CAD build for the part. Positions are in the model's coordinates, mm. Coordinates: 2 decimals unless noted, no trailing zeros. Loops run counter-clockwise (first coordinate to the right, second up) from the corner with the lowest first, then second, coordinate; pieces in that order, holes last. Notation, with made-up numbers: (18.5, 83) - (35.5, 83) arc R12 ccw to (35.5, 103) - close; hole circle Ø11 at (-24.75, 37.25). An arc over 180 degrees is marked (long way). Put each result on its own line as item: value.
```python
from build123d import *

# Parameters (mm, degrees)
CUT_EXTRUDE_1_DEPTH      = 10
PATTERN_CIRCULAR_2_COUNT = 28
SKETCH_3_R               = 5
CUT_EXTRUDE_2_DEPTH      = 26.454679665


with BuildPart() as part:
    # 草图1 → 旋转1 (revolve)
    with BuildSketch(Plane.XY, mode=Mode.PRIVATE) as revolve_1_sk:
        Polygon((-4.537524852, 10.783302268), (-14.537524852, 10.783302268), (-14.537524852, 1.783302268), (-15.787524852, 1.783302268), (-15.787524852, -3.216697732), (-3.287524852, -3.216697732), (-3.287524852, 1.783302268), (-4.537524852, 1.783302268), align=None)
    revolve(revolve_1_sk.sketch.rotate(Axis((-37.951477077, -3.216697732, 0), (1, 0, 0)), 90), axis=Axis((-37.951477077, -3.216697732, 0), (1, 0, 0)))

    # 草图2 → 切除-拉伸1 (cut)
    with BuildSketch(Plane.ZY.offset(14.537524852)):
        with BuildLine():
            Line((0.390901935, 85.320682721), (-0.569796452, 10.771702176))
            ThreePointArc((-0.569796452, 10.771702176), (0.830427689, 9.255687358), (2.419277547, 10.572685726))
            Line((2.419277547, 10.572685726), (11.35038276, 84.590986174))
            Line((11.35038276, 84.590986174), (21.256411219, 233.371913604))
            Line((21.256411219, 233.371913604), (10.296930394, 234.10161015))
            Line((10.296930394, 234.10161015), (0.390901935, 85.320682721))
        make_face()
    cut_extrude_1 = extrude(amount=-CUT_EXTRUDE_1_DEPTH, mode=Mode.SUBTRACT)

    # 阵列(圆周)2: 切除-拉伸1 ×28 about axis
    pattern_circular_2_axis = Axis((0, -3.216697732, 0), (1, 0, 0))
    for i in range(1, PATTERN_CIRCULAR_2_COUNT):
        add(cut_extrude_1.rotate(pattern_circular_2_axis, i * 360 / PATTERN_CIRCULAR_2_COUNT), mode=Mode.SUBTRACT)

    # 草图3 → 切除-拉伸2 (cut, through all)
    with BuildSketch(Plane.ZY.offset(15.787524852)):
        with Locations((0, -3.216697732)):
            Circle(SKETCH_3_R)
    extrude(amount=-CUT_EXTRUDE_2_DEPTH, mode=Mode.SUBTRACT)


solid = part.part
```
Q1. Slice it at A-A, the plane y = -1.25. Give the cut face in (x, z).
Determined:
outline: (-14.54, -12.88) - (-4.54, -12.88) - (-4.54, -4.6) - (-14.54, -4.6) - close; (-14.54, 4.6) - (-4.54, 4.6) - (-4.54, 12.34) - (-14.54, 12.34) - close
Q2. Mould opens along Z. For faces 1 (the flat face through (-4.538, -3, -6)), 2 (the cylindrical face through (-9.6, -14.8, 4.7)) say: +Z half, -Z half, draft (parallel to the pull), parting line (faces both ways), or undercut.
Determined:
face 1: draft
face 2: undercut
Q3. Wall check: L1, parallel to Z at x = -9, y = -2; L2, parallel to Y at x = -13.25, z = -4.5; L3, parallel to Y at x = -9.25, z = 0. Give the ranges that are in metal, low to high. Write a range as from..to.
Determined:
L1: -12.5..-4.85, 4.85..12.69
L2: -15.21..-5.4, -1.04..8.46
L3: -16.01..-8.22, 1.78..9.58
Q4. Pin check, flat tips, straight feed: pin 1 Ø4 at (x, z) = (-10.5, -9) entering from +Y; pin 2 Ø2 at (x, z) = (-13, -6) entering from +Y; pin 3 Ø1.5 at (y, z) = (-14.5, 8) entering from +X; pin 4 Ø11.5 at (y, z) = (-3.22, 0) entering from -X. Stop position of each tip, or through.
Determined:
pin 1: y = 7.36
pin 2: y = 9.14
pin 3: through
pin 4: x = -14.54
Q5. Slice it at B-B, the plane z = 0. Give the cut face in (x, y).
Determined:
outline: (-14.54, -16.01) - (-4.54, -16.01) - (-4.54, -8.22) - (-14.54, -8.22) - close; (-14.54, 1.78) - (-4.54, 1.78) - (-4.54, 9.58) - (-14.54, 9.58) - close
Q6. Slice it at C-C, the plane z = 7.25. Give the cut face in (x, y).
Determined:
outline: (-14.54, -13.41) - (-4.54, -13.41) - (-4.54, 7.51) - (-14.54, 7.51) - close
